CAD build for the part. Positions are in the model's coordinates, mm. A direction names the side the tool comes from. Coordinates: 2 decimals unless noted, no trailing zeros. Order: outer loops, then holes, each group sorted by start corner. A loop starts at its lowest first (then second) coordinate and runs counter-clockwise, first axis right, second up. Notation, with made-up numbers: M -33.75,67.25 L 12.25,67.25 A16 cw 12.25,79.25 Z; hole C 50,-12.75 d5. An arc over 180 degrees is marked long. One line per item, written item: value.
from build123d import *

# Parameters (mm, degrees)
F1_DEPTH = 8
F2_D     = 15
F3_D     = 15
F5_W     = 30
F5_H     = 4
F6_DEPTH = 30.001


with BuildPart() as f1:
    # F0 (on Front) → F1 (new body)
    with BuildSketch(Plane.XZ):
        with BuildLine():
            Line((188, 15), (0, 15))
            ThreePointArc((0, 15), (-15, 0), (0, -15))
            Line((0, -15), (188, -15))
            ThreePointArc((188, -15), (203, 0), (188, 15))
        make_face()
    extrude(amount=F1_DEPTH)

    # F2 (through all)
    with Locations(Plane(origin=(0, 0, 0), x_dir=(1, 0, 0), z_dir=(0, 1, 0))):
        with Locations((0, 0)):
            Hole(F2_D / 2)

    # F3 (through all)
    with Locations(Plane(origin=(0, 0, 0), x_dir=(1, 0, 0), z_dir=(0, 1, 0))):
        with Locations((188, 0)):
            Hole(F3_D / 2)

    # F5 (on offset) → F6 (cut, through all)
    with BuildSketch(Plane.XY.offset(15)):
        with Locations((0, -4.0625976841)):
            Rectangle(F5_W, F5_H)
    extrude(amount=-F6_DEPTH, mode=Mode.SUBTRACT)


solid = f1.part
Q1. Slice it at A-A (z = 0). List the corners of the cut face in (x, y), plus the area to 3 significant figures.
Recorded:
outline: M -15,-8 L -7.5,-8 L -7.5,-6.06 L -15,-6.06 Z; M -15,-2.06 L -7.5,-2.06 L -7.5,0 L -15,0 Z; M 7.5,-8 L 180.5,-8 L 180.5,0 L 7.5,0 L 7.5,-2.06 L 15,-2.06 L 15,-6.06 L 7.5,-6.06 Z; M 195.5,-8 L 203,-8 L 203,0 L 195.5,0 Z
area: 1,440 mm^2
Q2. Pin check, flat tips, straight feed: pin 1 Ø6 at (x, z) = (11.5, -11.5) entering from +Y; pin 2 Ø1.2 at (y, z) = (-5, -4) entering from -X; pin 3 Ø3 at (y, z) = (-1, 11) entering from -X. Stop position of each tip, or through.
Recorded:
pin 1: stops at y = 0
pin 2: stops at x = 15
pin 3: stops at x = -11.61
Q3. Slice it at C-C (z = -11). List the corners of the cut face in (x, y), plus the area to 3 significant figures.
Recorded:
outline: M -10.2,-8 L 198.2,-8 L 198.2,0 L -10.2,0 L -10.2,-2.06 L 15,-2.06 L 15,-6.06 L -10.2,-6.06 Z
area: 1,570 mm^2
Q4. Slice it at B-B (z = 11.5). List the corners of the cut face in (x, y).
Recorded:
outline: M -9.63,-8 L 197.63,-8 L 197.63,0 L -9.63,0 L -9.63,-2.06 L 15,-2.06 L 15,-6.06 L -9.63,-6.06 Z
Q5. Which spindle directions (+Z, -Z, +X, -X, +Y, -Y) get a long thin tool onto all of the face, cutting with end or side? Do faces 4 (the face through (93, -4, -15)), 5 (the face through (10, -2.063, 0)). Say none if no direction does.
Recorded:
face 4: -Z, +X, -X, +Y, -Y
face 5: +Z, -Z, -X
Q6. Drill centre lines: line 1 along Y through (x, z) = (-4, -9); line 2 along Z through (x, y) = (0, -1.6); line 3 along X through (y, z) = (-1.75, -1). Where is each one in solid material? Low to high.
Recorded:
line 1: y = -8 to -6.06, -2.06 to 0
line 2: z = -15 to -7.5, 7.5 to 15
line 3: x = -14.97 to -7.43, 7.43 to 180.57, 195.43 to 202.97
Q7. Mould opens along X. For faces 1 (the face through (95, -4, 15)), 2 (the face through (-15, -1, 0)), 3 (the face through (7.493, -1.046, -0.33)) say: released by +X, released by -X, zero draft, split by the parting line, or undercut.
Recorded:
face 1: zero draft
face 2: released by -X
face 3: undercut
